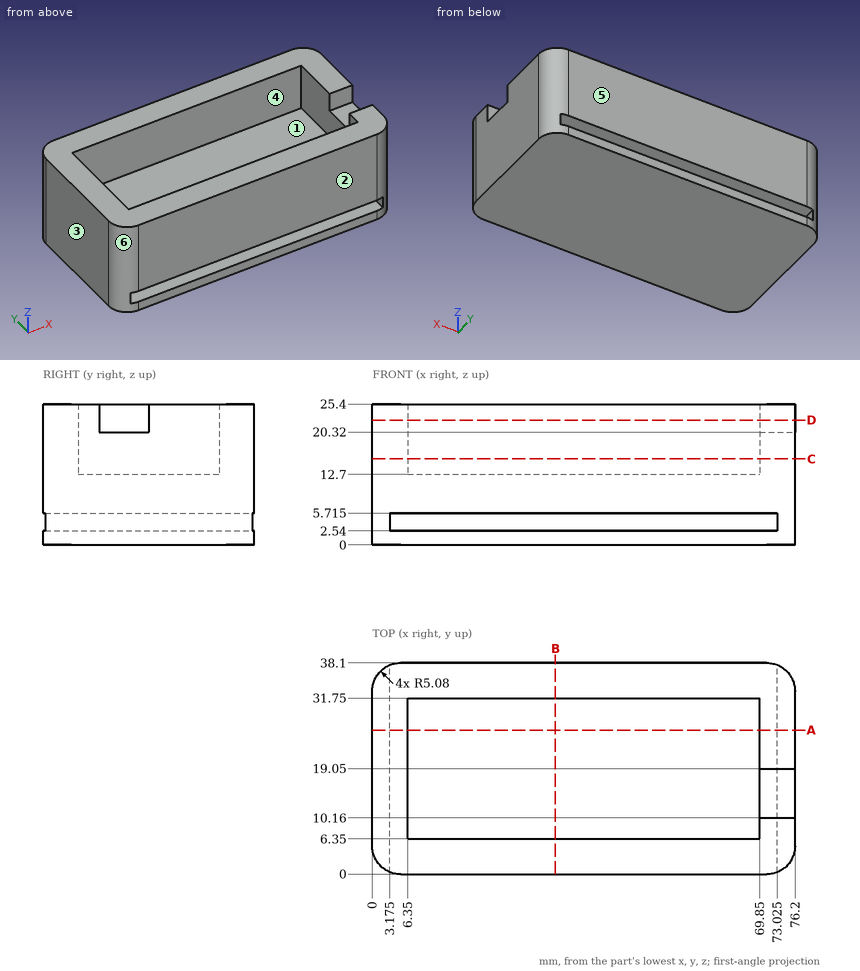
Here's the drawing with two shaded views (mm, measured from the low corner). I have some questions. A direction names the side the tool comes from. Give positions to 0.01 mm unless a question says otherwise; leave off trailing zeros. Write each loop counter-clockwise with the first axis right and the second up, starting at its lowest first coordinate (ties: lowest second). Pieces come first, ordered by that corner, then holes. Notation, with made-up numbers: (-17.75, -38.75) -> (18.25, -38.75) arc R21 ccw to (18.25, -24.75) -> close; hole circle Ø6 at (-12.75, 15). An arc over 180 degrees is marked (long way). Use one line per item in the form item = value. Start each with the question number.
1. Thinking about a two-plate mould opening in Y: for the marked faces 3, 4, 5 and 6, which applies, +Y half, -Y half, draft (parallel to the pull), parting line (faces both ways), or undercut?
2. Imagine slicing it at C-C on z = 15.5. List the corners of the cut face in (x, y) for me.
3. If I drill on L1, parallel to X at y = 22.5, z = 19; L2, parallel to Z at x = 42, y = 15 (3 decimals); L3, parallel to Y at x = 50, z = 17, over which ranges is the centre line in solid material (lowest first)?
4. Imagine slicing it at B-B on x = 33. List the corners of the cut face in (y, z) for me (3 decimals), plus the area to 3 significant figures.
5. On a 3-axis mill with a long thin cutter (end or side, diameter ignored), from which of +Z, -Z, +X, -X, +Y, -Y can I reach the whole of each face in a straight line? I mean the marked faces 1 and 2. Say none if no direction works.
6. Imagine slicing it at A-A on y = 26. List the corners of the cut face in (x, z) for me (3 decimals).
7. Imagine slicing it at D-D on z = 22.5. List the corners of the cut face in (x, y) for me, plus the area to 3 significant figures.
8. Will these pins go through, and if not, where does the flat tip stop? pin 1 Ø1.5 at (x, z) = (73, 22.5) entering from +Y; pin 2 Ø3 at (x, z) = (63, 3) entering from -Y; pin 3 Ø1 at (y, z) = (34, 17.5) entering from +X; pin 4 Ø7 at (x, y) = (73, 15) entering from +Z.
Entries:
q1.face_3 = draft
q1.face_4 = undercut
q1.face_5 = +Y half
q1.face_6 = -Y half
q2.outline = (0, 5.08) arc R5.08 ccw to (5.08, 0) -> (71.12, 0) arc R5.08 ccw to (76.2, 5.08) -> (76.2, 33.02) arc R5.08 ccw to (71.12, 38.1) -> (5.08, 38.1) arc R5.08 ccw to (0, 33.02) -> close; hole (6.35, 6.35) -> (69.85, 6.35) -> (69.85, 31.75) -> (6.35, 31.75) -> close
q3.L1 = 0 to 6.35, 69.85 to 76.2
q3.L2 = 0 to 2.54, 5.715 to 12.7
q3.L3 = 0 to 6.35, 31.75 to 38.1
q4.outline = (0, 0) -> (38.1, 0) -> (38.1, 2.54) -> (0, 2.54) -> close; (0, 5.715) -> (38.1, 5.715) -> (38.1, 25.4) -> (31.75, 25.4) -> (31.75, 12.7) -> (6.35, 12.7) -> (6.35, 25.4) -> (0, 25.4) -> close
q4.area = 524 mm²
q5.face_1 = +Z
q5.face_2 = +Z, -Z, +X, -X, -Y
q6.outline = (0, 0) -> (76.2, 0) -> (76.2, 25.4) -> (69.85, 25.4) -> (69.85, 12.7) -> (6.35, 12.7) -> (6.35, 25.4) -> (0, 25.4) -> close; hole (3.175, 2.54) -> (73.025, 2.54) -> (73.025, 5.715) -> (3.175, 5.715) -> close
q7.outline = (0, 5.08) arc R5.08 ccw to (5.08, 0) -> (71.12, 0) arc R5.08 ccw to (76.2, 5.08) -> (76.2, 10.16) -> (69.85, 10.16) -> (69.85, 6.35) -> (6.35, 6.35) -> (6.35, 31.75) -> (69.85, 31.75) -> (69.85, 19.05) -> (76.2, 19.05) -> (76.2, 33.02) arc R5.08 ccw to (71.12, 38.1) -> (5.08, 38.1) arc R5.08 ccw to (0, 33.02) -> close
q7.area = 1,210 mm²
q8.pin_1 = 37.97
q8.pin_2 = 0
q8.pin_3 = 76.18
q8.pin_4 = 20.32
